The figure shows three views and two pictorial views of one solid part (mm, origin at its lowest corner). Answer the questions. A direction names the side the tool comes from. Give positions to 0.01 mm unless a question says otherwise; leave off trailing zeros. Order: outer loops, then holes, each group sorted by start corner. A loop starts at its lowest first (then second) coordinate and runs counter-clockwise, first axis right, second up. Notation, with made-up numbers: (-9.75, 43.5) - (14.25, 43.5) arc R24 ccw to (14.25, 79.5) - close; hole circle Ø5 at (-30.5, 20.25). An arc over 180 degrees is marked (long way). Answer as a JSON object with one key per item and string values. Group by question number.
Q1. A cutting plane is placed at C-C, the plane y = 36.5. Give the vertices of the cut face in (x, z) (1 decimal).
Q2. Consider line 1 (Z direction, x = 37, y = 39); line 2 (X direction, y = 22.5, z = 9); line 3 (Y direction, x = 39, z = 4.75) (1 decimal). Determine where each line is inside the solid, lowest interval first.
Q3. Given pin 1 (10 mm diameter, centred on y = 39, z = 22.5, fed in from -X), flat-ended and moving along its own axis, determine where the tip first touches the part or whether it passes through.
Q4. For the marked faces 1, 2, 3 and 4, determine the directions among +Z, -Z, +X, -X, +Y, -Y from which every point of the face is accessible in a straight line to the end or side of a thin tool.
Q5. A cutting plane is placed at A-A, the plane x = 39. Give the vertices of the cut face in (y, z) (1 decimal), and give its area (3 significant figures).
Q6. A cutting plane is placed at B-B, the plane y = 20.5. Give the vertices of the cut face in (x, z).
Q7. A cutting plane is placed at D-D, the plane z = 4. Give the vertices of the cut face in (x, y) (1 decimal).
Q8. The mould has two halves that part along Y. Classify the marked faces 5, 6, 7 and 8: released by +Y, released by -Y, zero draft, split by the parting line, or undercut.
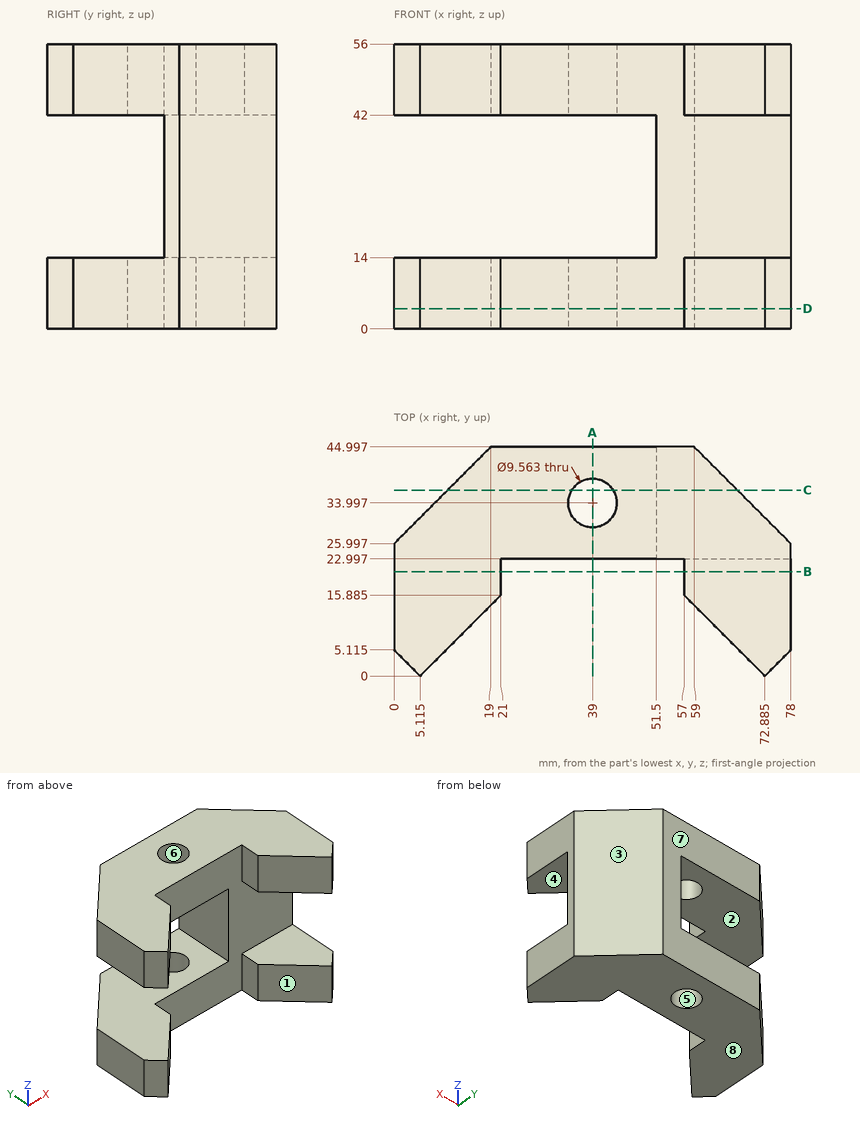
Reply:
{
 "1": {"outline": "(10.5, 0) - (34.9, 0) - (34.9, 14) - (10.5, 14) - close; (10.5, 42) - (34.9, 42) - (34.9, 56) - (10.5, 56) - close; (43.1, 0) - (67.5, 0) - (67.5, 56) - (43.1, 56) - (43.1, 42) - (51.5, 42) - (51.5, 14) - (43.1, 14) - close"},
 "2": {"line 1": "z = 0 to 14, 42 to 56", "line 2": "x = 0 to 21, 57 to 78", "line 3": "y = 23 to 29.2, 38.8 to 45"},
 "3": {"pin 1": "stops at x = 51.5"},
 "4": {"face 1": "+Z, -Z, -Y", "face 2": "-X, +Y, -Y", "face 3": "+Z, -Z, +X, +Y", "face 4": "+X, -X, -Y"},
 "5": {"outline": "(23, 0) - (29.2, 0) - (29.2, 14) - (23, 14) - close; (23, 42) - (29.2, 42) - (29.2, 56) - (23, 56) - close; (38.8, 0) - (45, 0) - (45, 14) - (38.8, 14) - close; (38.8, 42) - (45, 42) - (45, 56) - (38.8, 56) - close", "area": "348 mm^2"},
 "6": {"outline": "(0, 0) - (21, 0) - (21, 14) - (0, 14) - close; (0, 42) - (21, 42) - (21, 56) - (0, 56) - close; (57, 0) - (78, 0) - (78, 14) - (57, 14) - close; (57, 42) - (78, 42) - (78, 56) - (57, 56) - close"},
 "7": {"outline": "(0, 5.1) - (5.1, 0) - (21, 15.9) - (21, 23) - (57, 23) - (57, 15.9) - (72.9, 0) - (78, 5.1) - (78, 26) - (59, 45) - (19, 45) - (0, 26) - close; hole circle Ø9.6 at (39, 34)"},
 "8": {"face 5": "undercut", "face 6": "undercut", "face 7": "released by +Y", "face 8": "zero draft"}
}
